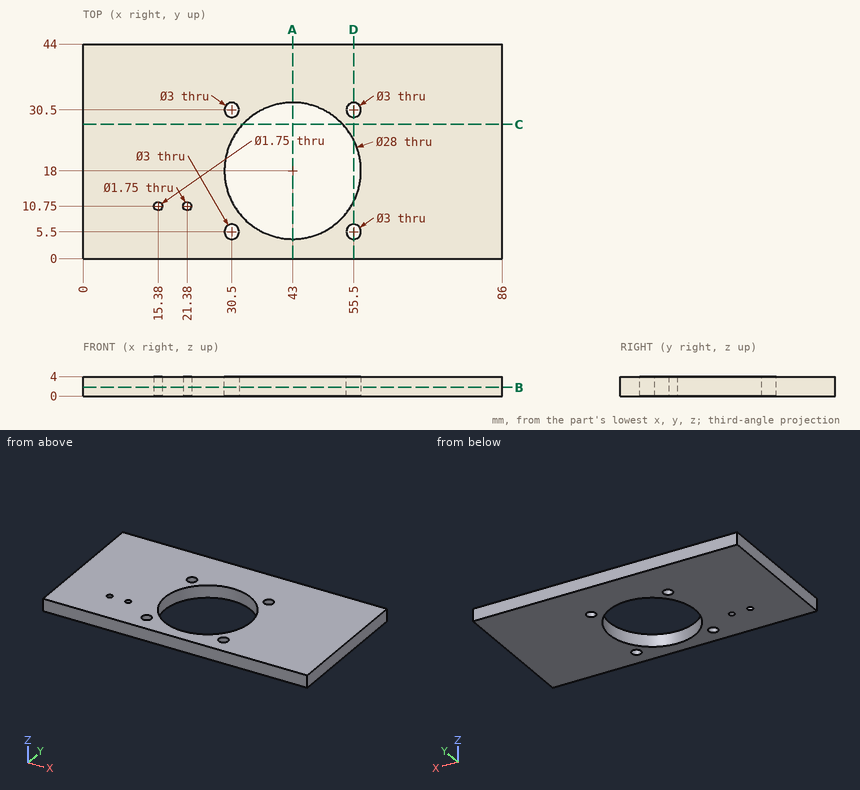
Input: dimensioned drawing with shaded views. Units: mm. Origin: part minimum x, y, z. Coordinates: 2 decimals unless noted, no trailing zeros. Order: outer loops, then holes, each group sorted by start corner. A loop starts at its lowest first (then second) coordinate and runs counter-clockwise, first axis right, second up. Notation, with made-up numbers: (27.5, -1) -> (58.5, -1) arc R15 cw to (58.5, 28) -> close; hole circle Ø9 at (-18, 71). An arc over 180 degrees is marked (long way). Answer in a Markdown table with one row per item.
Item 1: Ray query, L1, parallel to Y at x = 30.5, z = 1.9; L2, parallel to Y at x = 21.38, z = 1.25 (3 decimals); L3, parallel to X at y = 29.5, z = 1.85. Return the intervals inside material, ascending.
Return value:
| item | result |
|---|---|
| L1 | y = 0 to 4, 7 to 11.7, 24.3 to 29, 32 to 44 |
| L2 | y = 0 to 9.875, 11.625 to 44 |
| L3 | x = 0 to 29.38, 31.62 to 35.02, 50.98 to 54.38, 56.62 to 86 |
Item 2: Section D-D on x = 55.5. Output: boundary loops of the cut face in (y, z), plus the area to 3 significant figures.
Return value:
| item | result |
|---|---|
| outline | (0, 0) -> (4, 0) -> (4, 4) -> (0, 4) -> close; (7, 0) -> (11.7, 0) -> (11.7, 4) -> (7, 4) -> close; (24.3, 0) -> (29, 0) -> (29, 4) -> (24.3, 4) -> close; (32, 0) -> (44, 0) -> (44, 4) -> (32, 4) -> close |
| area | 102 mm² |
Item 3: Section C-C on y = 27.5. Output: boundary loops of the cut face in (x, z), plus the area to 3 significant figures.
Return value:
| item | result |
|---|---|
| outline | (0, 0) -> (32.72, 0) -> (32.72, 4) -> (0, 4) -> close; (53.28, 0) -> (86, 0) -> (86, 4) -> (53.28, 4) -> close |
| area | 262 mm² |
Item 4: Section B-B on z = 1.8. Output: boundary loops of the cut face in (x, y) (3 decimals).
Return value:
| item | result |
|---|---|
| outline | (0, 0) -> (86, 0) -> (86, 44) -> (0, 44) -> close; hole circle Ø1.75 at (15.38, 10.75); hole circle Ø1.75 at (21.38, 10.75); hole circle Ø3 at (30.5, 5.5); hole circle Ø28 at (43, 18); hole circle Ø3 at (30.5, 30.5); hole circle Ø3 at (55.5, 5.5); hole circle Ø3 at (55.5, 30.5) |
Item 5: Section A-A on x = 43. Output: boundary loops of the cut face in (y, z), plus the area to 3 significant figures.
Return value:
| item | result |
|---|---|
| outline | (0, 0) -> (4, 0) -> (4, 4) -> (0, 4) -> close; (32, 0) -> (44, 0) -> (44, 4) -> (32, 4) -> close |
| area | 64.0 mm² |
